The listing builds one solid part. Answer for the finished solid, in the listing's coordinates (mm). A direction names the side the tool comes from. Coordinates: 2 decimals unless noted, no trailing zeros. Order: outer loops, then holes, each group sorted by start corner. A loop starts at its lowest first (then second) coordinate and runs counter-clockwise, first axis right, second up. Notation, with made-up numbers: (88.5, 49.25) -> (137.5, 49.25) arc R31 ccw to (137.5, 87.25) -> close; hole circle Ø6 at (-23, 24). An arc over 180 degrees is marked (long way). Return JSON: item names as keys, results as strings.
```python
from build123d import *

# Parameters (mm, degrees)
F1_DEPTH = 5.08


with BuildPart() as f1:
    # F0 (on Right) → F1 (new body)
    with BuildSketch(Plane.YZ):
        Polygon((-35.573810339, 27.1448735148), (-35.573810339, 22.0602974296), (2.5212168694, 22.0602974296), (40.6162440777, 22.0602974296), (40.6162440777, 27.1448735148), align=None)
        Polygon((-39.6445272604, 19.0086872448), (-35.573810339, 22.0602974296), (-35.573810339, 27.1448735148), (-45.7443889554, 27.1448735148), align=None)
        Polygon((2.5212168694, -28.7568327039), (-35.573810339, 22.0602974296), (-39.6445272604, 19.0086872448), (-1.5472002365, -31.8067188336), align=None)
        Polygon((6.5896339752, -31.8067188336), (2.5212168694, -28.7568327039), (-1.5472002365, -31.8067188336), (2.5232048978, -37.2359524821), align=None)
        Polygon((40.6162440777, 22.0602974296), (2.5212168694, -28.7568327039), (6.5896339752, -31.8067188336), (44.6869609991, 19.0086872448), align=None)
        Polygon((40.6162440777, 27.1448735148), (40.6162440777, 22.0602974296), (44.6869609991, 19.0086872448), (50.7868226941, 27.1448735148), align=None)
    extrude(amount=F1_DEPTH)


solid = f1.part
```
Item 1: Which of the six approach directions +Z, -Z, +X, -X, +Y, -Y give full straight-line access (tool end or side, diameter ignored) to faces 4 (the flat face through (0, -1, 24)), 5 (the flat face through (3, 2, 22.06))?
Answer list:
{"face 4": "+Z, -Z, -X, +Y, -Y", "face 5": "+X, -X"}
Item 2: The part is cut by section B-B on y = -20.5. Determine the outline of the cut face in (x, z).
Answer list:
{"outline": "(0, -6.53) -> (5.08, -6.53) -> (5.08, 1.95) -> (0, 1.95) -> close; (0, 22.06) -> (5.08, 22.06) -> (5.08, 27.14) -> (0, 27.14) -> close"}
Item 3: A flat-ended cylindrical pin translates along its axis: pin 1 (2 mm diameter, centred on x = 2, z = -10, fed in from +Y). Find the tip coordinate at first contact, or state that the pin passes through.
Answer list:
{"pin 1": "y = 23.69"}
Item 4: The part is cut by section A-A on z = 17.5. Determine the outline of the cut face in (x, y).
Answer list:
{"outline": "(0, -38.51) -> (5.08, -38.51) -> (5.08, -32.16) -> (0, -32.16) -> close; (0, 37.2) -> (5.08, 37.2) -> (5.08, 43.56) -> (0, 43.56) -> close"}
Item 5: The part is cut by section C-C on x = 3.55. Determine the outline of the cut face in (y, z).
Answer list:
{"outline": "(-45.74, 27.14) -> (2.52, -37.24) -> (6.59, -31.81) -> (50.79, 27.14) -> close; hole (-35.57, 22.06) -> (2.52, -28.76) -> (40.62, 22.06) -> close"}
Item 6: Determine the mould class of faces 1 (the flat face through (2.504, 21.835, -2.993)), 2 (the flat face through (2.504, -16.26, -3.704)), 3 (the flat face through (3, 3, 27.145)) for opening direction Y: pulls with the +Y half, pulls with the -Y half, needs draft (parallel to the pull), parting line crosses it, or undercut.
Answer list:
{"face 1": "undercut", "face 2": "undercut", "face 3": "needs draft"}
Item 7: Find the intervals of material crossed by probe 1 along Y at (x, z) = (2.45, 11); probe 2 along Z at (x, y) = (2.1, -16.5); probe 3 along Z at (x, y) = (1.9, -17), in increasing order.
Answer list:
{"probe 1": "-33.64 to -27.28, 32.32 to 38.68", "probe 2": "-11.86 to -3.38, 22.06 to 27.14", "probe 3": "-11.2 to -2.72, 22.06 to 27.14"}
